Could you check a few things on this model? Use its own coordinates, in mm. Face numbers are marked on the shaded views. A direction names the side the tool comes from. Round coordinates to 2 decimals unless told otherwise and drop trailing zeros. Loops run counter-clockwise (first coordinate to the right, second up) from the corner with the lowest first, then second, coordinate; pieces in that order, holes last.
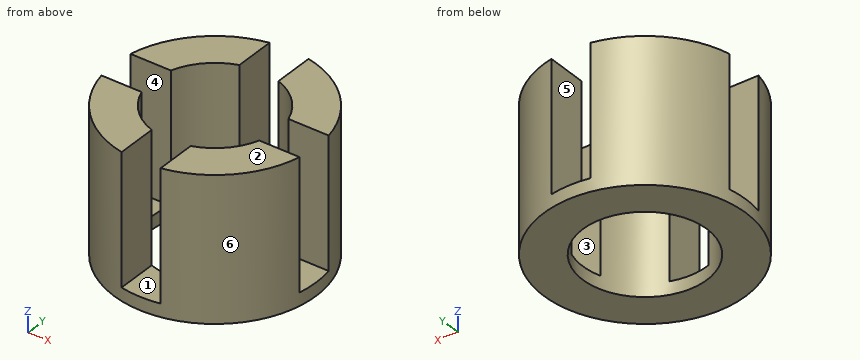
from build123d import *

# Parameters (mm, degrees)
F0_W     = 3
F0_H     = 11
F2_W     = 3
F2_H     = 5.261537
F2_W_2   = 5.261537
F2_H_2   = 3
F3_DEPTH = 10


with BuildPart() as f1:
    # F0 (on Front) → F1 (revolve)
    with BuildSketch(Plane.XZ):
        with Locations((-6.26, 28.5)):
            Rectangle(F0_W, F0_H)
    revolve(axis=Axis((0, 0, 29.352345), (0, 0, -1)))

    # F2 (on face) → F3 (cut)
    with BuildSketch(Plane.XY.offset(34)):
        with Locations((0, 6.592725)):
            Rectangle(F2_W, F2_H)
        with Locations((-6.592725, 0)):
            Rectangle(F2_W_2, F2_H_2)
        with Locations((0, -6.592725)):
            Rectangle(F2_W, F2_H)
        with Locations((6.592725, 0)):
            Rectangle(F2_W_2, F2_H_2)
    extrude(amount=-F3_DEPTH, mode=Mode.SUBTRACT)


solid = f1.part
Item 1: If we section it at C-C, the plane z = 27.5: Please give me the cut outline in (x, y).
Results list:
outline: (-7.61, -1.5) arc R7.76 ccw to (-1.5, -7.61) - (-1.5, -4.52) arc R4.76 cw to (-4.52, -1.5) - close; (-7.61, 1.5) - (-4.52, 1.5) arc R4.76 cw to (-1.5, 4.52) - (-1.5, 7.61) arc R7.76 ccw to start; (1.5, -7.61) arc R7.76 ccw to (7.61, -1.5) - (4.52, -1.5) arc R4.76 cw to (1.5, -4.52) - close; (1.5, 4.52) arc R4.76 cw to (4.52, 1.5) - (7.61, 1.5) arc R7.76 ccw to (1.5, 7.61) - close
Item 2: If I drill on line 1 along X through (y, z) = (-4.25, 27.25); line 2 along X through (y, z) = (-3.75, 27.5); line 3 along Y through (x, z) = (5.75, 27), over which ranges is the centre line in solid material (lowest first)?
Results list:
line 1: x = -6.49 to -2.14, 2.14 to 6.49
line 2: x = -6.79 to -2.93, 2.93 to 6.79
line 3: y = -5.21 to -1.5, 1.5 to 5.21
Item 3: For the marked faces 1, 2 and 3, which set-ups out of +Z, -Z, +X, -X, +Y, -Y let a thin tool reach every point of the face, with its end or its side?
Results list:
face 1: +Z, +Y, -Y
face 2: +Z, +X, -X, +Y, -Y
face 3: +Z, +X, -X
Item 4: Will these pins go through, and if not, where does the flat tip stop? pin 1 (3.5 mm diameter, centred on y = 6.5, z = 27, fed in from -X); pin 2 (4 mm diameter, centred on y = -1.5, z = 27.5, fed in from -X); pin 3 (1.5 mm diameter, centred on x = 0.5, y = 5.5, fed in from +Z).
Results list:
pin 1: stops at x = -6.14
pin 2: stops at x = -7.61
pin 3: stops at z = 24
Item 5: We'd pull the mould along X, two halves only. Please class the marked faces 4, 5 and 6: released by +X, released by -X, zero draft, split by the parting line, or undercut.
Results list:
face 4: zero draft
face 5: undercut
face 6: split by the parting line
Item 6: If we section it at A-A, the plane x = 0: Please give me the cut outline in (y, z), then the cut area to 3 significant figures.
Results list:
outline: (-7.76, 23) - (-4.76, 23) - (-4.76, 24) - (-7.76, 24) - close; (4.76, 23) - (7.76, 23) - (7.76, 24) - (4.76, 24) - close
area: 6.00 mm2
